Verification items for the finished model (mm, model axes). Face numbers are marked on the shaded views. A direction names the side the tool comes from. Give positions to 0.01 mm unless a question says otherwise; leave off trailing zeros. Order: outer loops, then holes, each group sorted by start corner. A loop starts at its lowest first (then second) coordinate and runs counter-clockwise, first axis right, second up. Notation, with made-up numbers: (71.25, 23.5) -> (109.25, 23.5) arc R14 cw to (109.25, 33.5) -> close; hole circle Ø7 at (89.25, 49.5). An arc over 180 degrees is marked (long way). One line per question, with ' | ' between items. Start each with the question number.
Q1. Material ranges on probe 1 along Z at (x, y) = (0, -33.25); probe 2 along Z at (x, y) = (0, -11); probe 3 along X at (y, z) = (12, 29), recorded low to high. Write a range as [from, to].
Q2. Access from +Z, -Z, +X, -X, +Y, -Y to the whole of each face (thin tool, end or side, straight path). Record for the marked faces 1, 2, 3 and 4.
Q3. Section check B-B on z = 29. Record the cut outline in (x, y).
Q4. Section check D-D on z = 12.5. Record the cut outline in (x, y), plus the area to 3 significant figures.
Q5. Section check C-C on x = 0. Record the cut outline in (y, z), plus the area to 3 significant figures.
Q6. Section check A-A on y = 2.5. Record the cut outline in (x, z), plus the area to 3 significant figures.
Q7. Go/stop test with flat-tipped pins: pin 1 (20 mm diameter, centred on x = -23, y = 15, fed in from +Z); pin 2 (18 mm diameter, centred on x = 0, z = 29, fed in from +Y); pin 3 (18 mm diameter, centred on x = 0, z = 29, fed in from -Y); pin 4 (10 mm diameter, centred on x = -11, z = 39, fed in from +Y). Record where each tip stops, or that it passes through.
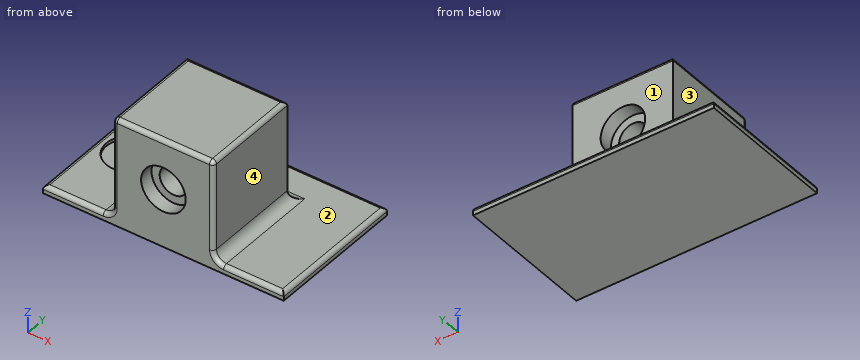
from build123d import *

# Parameters (mm, degrees)
SKETCH1_W           = 70
SKETCH1_H           = 120
BOSS_EXTRUDE1_DEPTH = 4
SKETCH2_W           = 50
SKETCH2_H           = 50
BOSS_EXTRUDE2_DEPTH = 50
SKETCH3_R           = 11.1
CUT_EXTRUDE1_DEPTH  = 7
SKETCH5_R           = 7
CUT_EXTRUDE3_DEPTH  = 103.396288995
CUT_EXTRUDE4_START  = -7
SKETCH6_R           = 11.1
CUT_EXTRUDE4_DEPTH  = 7
SKETCH7_R           = 12
CUT_EXTRUDE5_DEPTH  = 1.5
FILLET1_R           = 5
FILLET2_R           = 2


with BuildPart() as part:
    # Sketch1 → Boss-Extrude1 (new body)
    with BuildSketch(Plane(origin=(0, 0, 0), x_dir=(0, 1, 0), z_dir=(0, 0, 1))):
        Rectangle(SKETCH1_W, SKETCH1_H)
    extrude(amount=BOSS_EXTRUDE1_DEPTH)

    # Sketch2 → Boss-Extrude2 (add)
    with BuildSketch(Plane.XY.offset(4)):
        with Locations((0, -10)):
            Rectangle(SKETCH2_W, SKETCH2_H)
    extrude(amount=BOSS_EXTRUDE2_DEPTH)

    # Sketch3 → Cut-Extrude1 (cut)
    with BuildSketch(Plane.XZ.offset(35)):
        with Locations((0, 29)):
            Circle(SKETCH3_R)
    extrude(amount=-CUT_EXTRUDE1_DEPTH, mode=Mode.SUBTRACT)

    # Sketch5 → Cut-Extrude3 (cut, through all)
    with BuildSketch(Plane.XZ.offset(28)):
        with Locations((0, 29)):
            Circle(SKETCH5_R)
    extrude(amount=-CUT_EXTRUDE3_DEPTH, mode=Mode.SUBTRACT)

    # Sketch6 → Cut-Extrude4 (cut)
    with BuildSketch(Plane(origin=(0, 15, 0), x_dir=(-1, 0, 0), z_dir=(0, 1, 0)).offset(CUT_EXTRUDE4_START)):
        with Locations(Location((0, 29, 0), (0, 0, 180))):
            Circle(SKETCH6_R)
    extrude(amount=CUT_EXTRUDE4_DEPTH, mode=Mode.SUBTRACT)

    # Sketch7 → Cut-Extrude5 (cut)
    with BuildSketch(Plane.XY.offset(4)):
        with Locations((-44, 2.5)):
            Circle(SKETCH7_R)
    extrude(amount=-CUT_EXTRUDE5_DEPTH, mode=Mode.SUBTRACT)

    # Fillet1
    fillet1_edges = [part.edges().sort_by_distance(p)[0] for p in [
        (25, -10, 4),
        (0, 15, 4),
        (-25, -10, 4),
    ]]
    fillet(fillet1_edges, radius=FILLET1_R)

    # Fillet2
    fillet2_edges = [part.edges().sort_by_distance(p)[0] for p in [
        (-45, -35, 4),
        (25, -35, 31.5),
        (60, 0, 4),
        (-25, -35, 31.5),
        (25, -10, 54),
        (0, 15, 54),
        (-25, -10, 54),
        (0, -35, 54),
        (0, 35, 4),
        (45, -35, 4),
        (26.464466094, -35, 5.464466094),
        (-26.464466094, -35, 5.464466094),
        (-60, 0, 4),
    ]]
    fillet(fillet2_edges, radius=FILLET2_R)


solid = part.part
Filled in:
1) probe 1: [0, 17.9], [40.1, 53.98] | probe 2: [0, 22], [36, 54] | probe 3: [-25, -11.1], [11.1, 25]
2) face 1: +Z, +X, -X, +Y | face 2: +Z, +Y | face 3: +Z, -X, +Y, -Y | face 4: +Z, +X, +Y, -Y
3) outline: (-25, -33) arc R2 ccw to (-23, -35) -> (-11.1, -35) -> (-11.1, -28) -> (-7, -28) -> (-7, 8) -> (-11.1, 8) -> (-11.1, 15) -> (-25, 15) -> close; (7, -28) -> (11.1, -28) -> (11.1, -35) -> (23, -35) arc R2 ccw to (25, -33) -> (25, 15) -> (11.1, 15) -> (11.1, 8) -> (7, 8) -> close
4) outline: (-25, -33) arc R2 ccw to (-23, -35) -> (23, -35) arc R2 ccw to (25, -33) -> (25, 15) -> (-25, 15) -> close | area: 2,500 mm²
5) outline: (-35, 0) -> (35, 0) -> (35, 2) arc R2 ccw to (33, 4) -> (20, 4) arc R5 cw to (15, 9) -> (15, 17.9) -> (8, 17.9) -> (8, 22) -> (-28, 22) -> (-28, 17.9) -> (-35, 17.9) -> close; (-35, 40.1) -> (-28, 40.1) -> (-28, 36) -> (8, 36) -> (8, 40.1) -> (15, 40.1) -> (15, 52) arc R2 ccw to (13, 54) -> (-33, 54) arc R2 ccw to (-35, 52) -> close | area: 1,970 mm²
6) outline: (-60, 0) -> (60, 0) -> (60, 2) arc R2 ccw to (58, 4) -> (30, 4) arc R5 cw to (25, 9) -> (25, 52) arc R2 ccw to (23, 54) -> (-23, 54) arc R2 ccw to (-25, 52) -> (-25, 9) arc R5 cw to (-30, 4) -> (-32, 4) -> (-32, 2.5) -> (-56, 2.5) -> (-56, 4) -> (-58, 4) arc R2 ccw to (-60, 2) -> close; hole circle Ø14 at (0, 29) | area: 2,800 mm²
7) pin 1: z = 54 | pin 2: y = 8 | pin 3: y = -28 | pin 4: y = 15
